Build history of the part. All positions in model axes, mm. A direction names the side the tool comes from. Round coordinates to 2 decimals unless told otherwise and drop trailing zeros. Write each loop counter-clockwise with the first axis right and the second up, starting at its lowest first coordinate (ties: lowest second). Pieces come first, ordered by that corner, then holes.
1) Wall check: probe 1 along Y at (x, z) = (-3, 23.5); probe 2 along X at (y, z) = (-18, 1.75). Give the ranges that are in metal, low to high.
2) Saw through at C-C (z = 14). Write the cut outline in (x, y).
3) Pull direction Y, two halves, no side cores. Call faces 3 (the flat face through (0, 11, 0)), 4 (the flat face through (0, -7.5, 22)), 5 (the flat face through (0, -25, 22)), 6 (the flat face through (0, 25, 22)): +Y half, -Y half, draft (parallel to the pull), parting line (faces both ways), or undercut.
4) Which spindle directions (+Z, -Z, +X, -X, +Y, -Y) get a long thin tool onto all of the face, cutting with end or side? Do faces 1 (the flat face through (25, 0, 22)), 2 (the flat face through (7.5, 0, 22)). Say none if no direction does.
5) Saw through at A-A (y = -5). Write the cut outline in (x, z), plus the area to 4 significant figures.
from build123d import *

# Parameters (mm, degrees)
F0_W     = 50
F0_H     = 50
F0_W_2   = 15
F0_H_2   = 15
F1_DEPTH = 45
F3_DEPTH = 25


with BuildPart() as f1:
    # F0 (on Top) → F1 (new body)
    with BuildSketch(Plane.XY):
        Rectangle(F0_W, F0_H)
        Rectangle(F0_W_2, F0_H_2, mode=Mode.SUBTRACT)
    extrude(amount=F1_DEPTH)

    # F2 (on face) → F3 (cut)
    with BuildSketch(Plane.XZ.offset(25)):
        with BuildLine():
            ThreePointArc((2.4366985862, 0), (2.8557044454, 0.8307872277), (3, 1.75))
            ThreePointArc((3, 1.75), (-0.9192127723, 4.6057044454), (-2.4366985862, 0))
            Line((-2.4366985862, 0), (2.4366985862, 0))
        make_face()
    extrude(amount=-F3_DEPTH, mode=Mode.SUBTRACT)


solid = f1.part
Evaluation:
1. probe 1: y = -25 to -7.5, 7.5 to 25
1. probe 2: x = -25 to -3, 3 to 25
2. outline: (-25, -25) - (25, -25) - (25, 25) - (-25, 25) - close; hole (-7.5, -7.5) - (7.5, -7.5) - (7.5, 7.5) - (-7.5, 7.5) - close
3. face 3: draft
3. face 4: undercut
3. face 5: -Y half
3. face 6: +Y half
4. face 1: +Z, -Z, +X, +Y, -Y
4. face 2: +Z, -Z
5. outline: (-25, 0) - (-7.5, 0) - (-7.5, 45) - (-25, 45) - close; (7.5, 0) - (25, 0) - (25, 45) - (7.5, 45) - close
5. area: 1,575 mm2
